```python
from build123d import *

# Parameters (mm, degrees)
BOSS_EXTRUDE1_DEPTH = 317.5
FILLET1_R           = 6.35
SKETCH3_R           = 2.38125
CUT_EXTRUDE1_DEPTH  = 317.5
SKETCH4_R           = 2.38125
CUT_EXTRUDE2_DEPTH  = 317.5
LPATTERN5_COUNT     = 4
LPATTERN5_PITCH     = 100.0125


with BuildPart() as part:
    # Sketch1 → Boss-Extrude1 (new body)
    with BuildSketch(Plane.XY):
        Polygon((75.565, 0), (-75.565, 0), (-90.065, 3.13), (-90.904357489, -0.758397314), (-72.355, -4.7625), (72.355, -4.7625), (90.904357489, -0.758397314), (90.065, 3.13), align=None)
    extrude(amount=BOSS_EXTRUDE1_DEPTH)

    # Fillet1
    fillet1_edges = [part.edges().sort_by_distance(p)[0] for p in [
        (-90.484678745, 1.185801343, 0),
        (90.484678745, 1.185801343, 317.5),
        (-90.484678745, 1.185801343, 317.5),
        (90.484678745, 1.185801343, 0),
    ]]
    fillet(fillet1_edges, radius=FILLET1_R)

    # Sketch3 → Cut-Extrude1 (cut)
    with BuildSketch(Plane(origin=(-3.364295287, -15.5853935, 0), x_dir=(0.977485615, -0.211002067, 0), z_dir=(0.211002067, 0.977485615, 0))):
        with Locations((-81.280689445, -9.525)):
            Circle(SKETCH3_R)
        with Locations((-81.280689445, -122.2375)):
            Circle(SKETCH3_R)
        with Locations((-81.280689445, -209.55)):
            Circle(SKETCH3_R)
        with Locations((-81.280689445, -309.5625)):
            Circle(SKETCH3_R)
    extrude(amount=-CUT_EXTRUDE1_DEPTH, mode=Mode.SUBTRACT)

    # Sketch4 → Cut-Extrude2 (cut)
    with BuildSketch(Plane(origin=(3.364295287, -15.5853935, 0), x_dir=(0.977485615, 0.211002067, 0), z_dir=(-0.211002067, 0.977485615, 0))):
        with Locations((81.280689445, -9.525)):
            Circle(SKETCH4_R)
    cut_extrude2 = extrude(amount=-CUT_EXTRUDE2_DEPTH, mode=Mode.SUBTRACT)

    # LPattern5: Cut-Extrude2 ×4
    with Locations(*[(0, 0, i * LPATTERN5_PITCH) for i in range(1, LPATTERN5_COUNT)]):
        add(cut_extrude2, mode=Mode.SUBTRACT)


solid = part.part
```
Work out the finished part from the listing and answer in its coordinate system (mm). A direction names the side the tool comes from. Give positions to 0.01 mm unless a question says otherwise; leave off trailing zeros. Write each loop counter-clockwise with the first axis right and the second up, starting at its lowest first coordinate (ties: lowest second). Pieces come first, ordered by that corner, then holes.
(1) Which of the six approach directions +Z, -Z, +X, -X, +Y, -Y give full straight-line access (tool end or side, diameter ignored) to faces 1 (the cylindrical face through (-88.72, 0.78, 315.59)), 2 (the flat face through (82.916, 1.587, 156.528))?
Final values:
face 1: +Z, -X, +Y
face 2: +Z, -Z, +Y
(2) Straight lines are drawn through the part: line 1 (Y direction, x = 54.5, z = 284); line 2 (Y direction, x = -81.5, z = 197). For each, find the intervals that lie inside material, in ascending order.
Final values:
line 1: y = -4.76 to 0
line 2: y = -2.79 to 1.28
(3) Flat-ended cylindrical pins translate along their axes: pin 1 Ø12 at (x, z) = (8, 113.5) entering from +Y; pin 2 Ø2 at (y, z) = (1.5, 179) entering from +X; pin 3 Ø2 at (y, z) = (-0.5, 154) entering from -X; pin 4 Ø3 at (y, z) = (0, 268) entering from +X. Find the tip coordinate at first contact, or state that the pin passes through.
Final values:
pin 1: stops at y = 0
pin 2: stops at x = 90.63
pin 3: stops at x = -90.9
pin 4: stops at x = 90.9
(4) The mould has two halves that part along X. Classify faces 3 (the flat face through (-81.76, -2.732, 156.528)), 4 (the flat face through (1, 0, 157)), 5 (the flat face through (-1, -2, 0)), 6 (the flat face through (81.5, -2.79, 156.53)): pulls with the +X half, pulls with the -X half, needs draft (parallel to the pull), parting line crosses it, or undercut.
Final values:
face 3: pulls with the -X half
face 4: undercut
face 5: needs draft
face 6: pulls with the +X half
(5) The part is cut by section B-B on x = 63. Write down the section's boundary in (y, z), plus the area to 3 significant figures.
Final values:
outline: (-4.76, 0) - (0, 0) - (0, 317.5) - (-4.76, 317.5) - close
area: 1,510 mm2
(6) The part is cut by section A-A on z = 281. Write down the section's boundary in (x, y) (1 decimal), plus the area to 3 significant figures.
Final values:
outline: (-90.9, -0.8) - (-72.4, -4.8) - (72.4, -4.8) - (90.9, -0.8) - (90.1, 3.1) - (75.6, 0) - (-75.6, 0) - (-90.1, 3.1) - close
area: 839 mm2
